Input: part model. Units: mm. Frame: model coordinates. Face numbers are marked on the shaded views. A direction names the side the tool comes from. Coordinates: 2 decimals unless noted, no trailing zeros. Loops run counter-clockwise (first coordinate to the right, second up) from the corner with the lowest first, then second, coordinate; pieces in that order, holes last. Notation, with made-up numbers: M -28,53.25 L 0,53.25 A30 cw 0,75.25 Z; hole C 6,8.5 d9. An arc over 180 degrees is marked long. Use a Markdown table: item, result. Add a question column.
1. Section A-A on z = 3.75. State how many separate pieces and enclosed holes the cut face has, then the cut area to 3 significant figures.
2. Section B-B on x = -5. Output: boundary loops of the cut face in (y, z), then the cut area to 3 significant figures.
3. Section C-C on y = 19.5. Output: boundary loops of the cut face in (x, z).
4. Section D-D on x = 21.5. Output: boundary loops of the cut face in (y, z), then the cut area to 3 significant figures.
5. Line query: L1, parallel to X at y = -41, z = 8.75; L2, parallel to X at y = 9, z = 5; L3, parallel to X at y = 29.5, z = 8.25. Output: solid intervals per line, ascending. Write a range as [from, to].
6. Draft query along Y for the marked faces 3, 4 and 5. Return one class per face: +Y half, -Y half, draft (parallel to the pull), parting line (faces both ways), or undercut.
7. Pin query (flat end, axial travel): pin 1 (5 mm diameter, centred on x = 28.5, y = 0.5, fed in from +Z); pin 2 (11.5 mm diameter, centred on x = 4, y = -13, fed in from +Z); pin 3 (3.5 mm diameter, centred on x = -35, y = 45.5, fed in from +Z). Return the tip coordinate at first contact, or that it passes through.
8. Set-up query: the marked faces 1 and 2. Return all of +Z, -Z, +X, -X, +Y, -Y with unobstructed straight access to the full face (end or side cutting, diameter ignored); none if empty.
```python
from build123d import *

# Parameters (mm, degrees)
F0_W      = 87
F0_H      = 115
F1_DEPTH  = 2
F3_DEPTH  = 10
F2_R      = 3
F4_DEPTH  = 7
F5_DEPTH  = 7
F7_DEPTH  = 25
F8_DEPTH  = 6
F6_W      = 5
F6_H      = 5.0000016391
F6_H_2    = 4.9999983609
F6_H_3    = 4.999999553
F6_H_4    = 5.000000447
F9_DEPTH  = 25
F6_W_2    = 3
F10_DEPTH = 5
F2_W      = 15
F2_H      = 18
F11_DEPTH = 1
F6_W_3    = 2
F12_DEPTH = 5
F6_H_5    = 4.9999998137
F13_DEPTH = 5


with BuildPart() as f1:
    # F0 (on Top) → F1 (new body)
    with BuildSketch(Plane.XY):
        Rectangle(F0_W, F0_H)
    extrude(amount=F1_DEPTH)

    # F2 (on face) → F3 (join)
    with BuildSketch(Plane.XY.offset(2)):
        Polygon((33.5, -54.5), (-33.5, -54.5), (-33.5, 39.5), (-33.5, 57.5), (-43.5, 57.5), (-43.5, -57.5), (43.5, -57.5), (43.5, 57.5), (33.5, 57.5), (33.5, 39.5), align=None)
    extrude(amount=F3_DEPTH)

    # F2 (on face) → F4 (join)
    with BuildSketch(Plane.XY.offset(2)):
        with Locations((0, -44.5)):
            Circle(F2_R)
    extrude(amount=F4_DEPTH)

    # F2 (on face) → F5 (join)
    with BuildSketch(Plane.XY.offset(2)):
        Polygon((11.5, 39.5), (-11.5, 39.5), (-11.5, 6.5), (-6.5, 6.5), (-6.5, 1.5), (-11.5, 1.5), (-11.5, -32.5), (11.5, -32.5), (11.5, 1.5), (6.5, 1.5), (6.5, 6.5), (11.5, 6.5), align=None)
    extrude(amount=F5_DEPTH)

    # F2 (on face) → F7 (cut)
    with BuildSketch(Plane.XY.offset(2)):
        Polygon((-18.5, 57.5), (-18.5, 39.5), (-11.5, 39.5), (11.5, 39.5), (18.5, 39.5), (18.5, 57.5), align=None)
    extrude(amount=-F7_DEPTH, mode=Mode.SUBTRACT)

    # F6 (on face) → F8 (cut)
    with BuildSketch(Plane.XY.offset(12)):
        Polygon((41.5, -12.5000001863), (41.5, 32.5), (36.5, 32.5), (36.5, -12.5000001863), (36.5, -17.5), (36.5, -47.5), (41.5, -47.5), (41.5, -17.5), align=None)
    extrude(amount=-F8_DEPTH, mode=Mode.SUBTRACT)

    # F6 (on face) → F9 (cut)
    with BuildSketch(Plane.XY.offset(12)):
        Polygon((-40.5, 47.5), (-40.5, 42.500000447), (-40.5, 37.5), (-36.5, 37.5), (-36.5, 42.500000447), (-36.5, 47.5), (-36.5, 57.5), (-40.5, 57.5), align=None)
        with Locations((39, 54.9999991804)):
            Rectangle(F6_W, F6_H)
        with Locations((39, 49.9999991804)):
            Rectangle(F6_W, F6_H_2)
        with Locations((39, 45.0000002235)):
            Rectangle(F6_W, F6_H_3)
        with Locations((39, 40.0000002235)):
            Rectangle(F6_W, F6_H_4)
    extrude(amount=-F9_DEPTH, mode=Mode.SUBTRACT)

    # F6 (on face) → F10 (cut)
    with BuildSketch(Plane.XY.offset(12)):
        with Locations((-42, 45.0000002235)):
            Rectangle(F6_W_2, F6_H_3)
        with Locations((-35, 45.0000002235)):
            Rectangle(F6_W_2, F6_H_3)
    extrude(amount=-F10_DEPTH, mode=Mode.SUBTRACT)

    # F2 (on face) → F11 (cut)
    with BuildSketch(Plane.XY.offset(2)):
        with Locations((-26, 48.5)):
            Rectangle(F2_W, F2_H)
        with Locations((26, 48.5)):
            Rectangle(F2_W, F2_H)
    extrude(amount=-F11_DEPTH, mode=Mode.SUBTRACT)

    # F6 (on face) → F12 (cut)
    with BuildSketch(Plane.XY.offset(12)):
        with Locations((35, 45.0000002235)):
            Rectangle(F6_W_2, F6_H_3)
        with Locations((42.5, 45.0000002235)):
            Rectangle(F6_W_3, F6_H_3)
    extrude(amount=-F12_DEPTH, mode=Mode.SUBTRACT)

    # F6 (on face) → F13 (cut)
    with BuildSketch(Plane.XY.offset(12)):
        with Locations((35, -15.0000000931)):
            Rectangle(F6_W_2, F6_H_5)
        with Locations((42.5, -15.0000000931)):
            Rectangle(F6_W_3, F6_H_5)
    extrude(amount=-F13_DEPTH, mode=Mode.SUBTRACT)


solid = f1.part
```
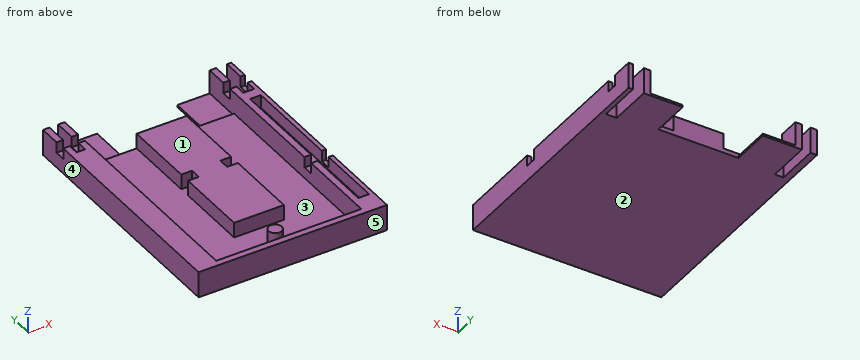
Answers below:
| question | item | result |
|---|---|---|
| 1 | separate pieces | 3 |
| 1 | enclosed holes | 0 |
| 1 | area | 3,960 mm² |
| 2 | outline | M -57.5,0 L 39.5,0 L 39.5,9 L -32.5,9 L -32.5,2 L -54.5,2 L -54.5,12 L -57.5,12 Z |
| 2 | area | 728 mm² |
| 3 | outline | M -43.5,0 L 43.5,0 L 43.5,12 L 41.5,12 L 41.5,6 L 36.5,6 L 36.5,12 L 33.5,12 L 33.5,2 L 11.5,2 L 11.5,9 L -11.5,9 L -11.5,2 L -33.5,2 L -33.5,12 L -43.5,12 Z |
| 4 | outline | M -57.5,0 L 57.5,0 L 57.5,1 L 39.5,1 L 39.5,2 L -54.5,2 L -54.5,12 L -57.5,12 Z |
| 4 | area | 242 mm² |
| 5 | L1 | x = [-43.5, -33.5], [33.5, 36.5], [41.5, 43.5] |
| 5 | L2 | x = [-43.5, -33.5], [-11.5, 11.5], [33.5, 43.5] |
| 5 | L3 | x = [-43.5, -33.5], [-11.5, 11.5], [33.5, 36.5], [41.5, 43.5] |
| 6 | face 3 | undercut |
| 6 | face 4 | draft |
| 6 | face 5 | -Y half |
| 7 | pin 1 | stops at z = 2 |
| 7 | pin 2 | stops at z = 9 |
| 7 | pin 3 | stops at z = 7 |
| 8 | face 1 | +Z, +Y |
| 8 | face 2 | -Z, +X, -X, +Y, -Y |
